The listing builds one solid part. Answer for the finished solid, in the listing's coordinates (mm). Give positions to 0.01 mm unless a question says otherwise; leave off trailing zeros. Write each loop counter-clockwise with the first axis right and the second up, starting at its lowest first coordinate (ties: lowest second). Pieces come first, ordered by that corner, then holes. Notation, with made-up numbers: M 47.25,44.5 L 93.25,44.5 A25 cw 93.25,56.5 Z; hole C 89.25,-4 d9. An arc over 180 degrees is marked long. Return JSON: item names as keys, results as strings.
from build123d import *

# Parameters (mm, degrees)
SKETCH1_W           = 38.1
SKETCH1_H           = 711.2
BOSS_EXTRUDE1_DEPTH = 3.175
FILLET1_R           = 2.54
SKETCH2_R           = 6.35
CUT_EXTRUDE1_DEPTH  = 4.175


with BuildPart() as part:
    # Sketch1 → Boss-Extrude1 (new body)
    with BuildSketch(Plane(origin=(0, 0, 0), x_dir=(1, 0, 0), z_dir=(0, 1, 0))):
        with Locations((19.05, 355.6)):
            Rectangle(SKETCH1_W, SKETCH1_H)
    extrude(amount=BOSS_EXTRUDE1_DEPTH)

    # Fillet1
    fillet1_edges = [part.edges().sort_by_distance(p)[0] for p in [
        (38.1, 1.5875, -711.2),
        (38.1, 1.5875, 0),
    ]]
    fillet(fillet1_edges, radius=FILLET1_R)

    # Sketch2 → Cut-Extrude1 (cut, through all)
    with BuildSketch(Plane(origin=(0, 3.175, 0), x_dir=(1, 0, 0), z_dir=(0, 1, 0))):
        with Locations((25.4, 660.4)):
            Circle(SKETCH2_R)
        with Locations((25.4, 457.2)):
            Circle(SKETCH2_R)
        with Locations((25.4, 254)):
            Circle(SKETCH2_R)
        with Locations((25.4, 50.8)):
            Circle(SKETCH2_R)
    extrude(amount=-CUT_EXTRUDE1_DEPTH, mode=Mode.SUBTRACT)


solid = part.part
Item 1: Find the intervals of material crossed by line 1 (Z direction, x = 25.4, y = 2); line 2 (X direction, y = 2, z = -254); line 3 (Z direction, x = 21, y = 0.95), in increasing order.
Geometry results:
{"line 1": "z = -711.2 to -666.75, -654.05 to -463.55, -450.85 to -260.35, -247.65 to -57.15, -44.45 to 0", "line 2": "x = 0 to 19.05, 31.75 to 38.1", "line 3": "z = -711.2 to -664.98, -655.82 to -461.78, -452.62 to -258.58, -249.42 to -55.38, -46.22 to 0"}
Item 2: A cutting plane is placed at A-A, the plane x = 25.4. Write down the section's boundary in (y, z) (3 decimals).
Geometry results:
{"outline": "M 0,-711.2 L 3.175,-711.2 L 3.175,-666.75 L 0,-666.75 Z; M 0,-654.05 L 3.175,-654.05 L 3.175,-463.55 L 0,-463.55 Z; M 0,-450.85 L 3.175,-450.85 L 3.175,-260.35 L 0,-260.35 Z; M 0,-247.65 L 3.175,-247.65 L 3.175,-57.15 L 0,-57.15 Z; M 0,-44.45 L 3.175,-44.45 L 3.175,0 L 0,0 Z"}
Item 3: Determine the mould class of faces 1 (the cylindrical face through (24.6, 1.6, -666.7)), 2 (the flat face through (19, 3.175, -361)) for opening direction Z: +Z half, -Z half, draft (parallel to the pull), parting line (faces both ways), or undercut.
Geometry results:
{"face 1": "undercut", "face 2": "draft"}
Item 4: A cutting plane is placed at C-C, the plane y = 1.1. Write down the section's boundary in (x, z), plus the area to 3 significant figures.
Geometry results:
{"outline": "M 0,-711.2 L 35.56,-711.2 A2.54 ccw 38.1,-708.66 L 38.1,-2.54 A2.54 ccw 35.56,0 L 0,0 Z; hole C 25.4,-660.4 d12.7; hole C 25.4,-457.2 d12.7; hole C 25.4,-254 d12.7; hole C 25.4,-50.8 d12.7", "area": "26,600 mm2"}
Item 5: A cutting plane is placed at B-B, the plane z = -50.8. Write down the section's boundary in (x, y) (3 decimals), plus the area to 3 significant figures.
Geometry results:
{"outline": "M 0,0 L 19.05,0 L 19.05,3.175 L 0,3.175 Z; M 31.75,0 L 38.1,0 L 38.1,3.175 L 31.75,3.175 Z", "area": "80.6 mm2"}
